```python
from build123d import *

# Parameters (mm, degrees)
SKIZZE1_W                       = 12
SKIZZE1_H                       = 29
SKIZZE1_W_2                     = 15
SKIZZE1_H_2                     = 4
AUFSATZ_LINEAR_AUSTRAGEN1_DEPTH = 4
SKIZZE2_W                       = 1.5
SKIZZE2_H                       = 4
SCHNITT_LINEAR_AUSTRAGEN1_DEPTH = 5
VERRUNDUNG1_R                   = 2


with BuildPart() as part:
    # Skizze1 → Aufsatz-Linear austragen1 (new body)
    with BuildSketch(Plane.XY):
        with Locations((0, -16.5)):
            Rectangle(SKIZZE1_W, SKIZZE1_H)
        Rectangle(SKIZZE1_W_2, SKIZZE1_H_2)
    extrude(amount=AUFSATZ_LINEAR_AUSTRAGEN1_DEPTH)

    # Skizze2 → Schnitt-Linear austragen1 (cut, through all)
    with BuildSketch(Plane.XY.offset(4)):
        with Locations((-5.25, -24)):
            Rectangle(SKIZZE2_W, SKIZZE2_H)
        with Locations((5.25, -24)):
            Rectangle(SKIZZE2_W, SKIZZE2_H)
    extrude(amount=-SCHNITT_LINEAR_AUSTRAGEN1_DEPTH, mode=Mode.SUBTRACT)

    # Verrundung1
    verrundung1_edges = [part.edges().sort_by_distance(p)[0] for p in [
        (6, -31, 2),
        (-6, -31, 2),
    ]]
    fillet(verrundung1_edges, radius=VERRUNDUNG1_R)


solid = part.part
```
Geometry: final body of the model. Coordinates: model frame, mm. A direction names the side the tool comes from. Round coordinates to 2 decimals unless told otherwise and drop trailing zeros. Loops run counter-clockwise (first coordinate to the right, second up) from the corner with the lowest first, then second, coordinate; pieces in that order, holes last.
Item 1: Section B-B, the plane y = -17. Output: boundary loops of the cut face in (x, z).
Checked values:
outline: (-6, 0) - (6, 0) - (6, 4) - (-6, 4) - close
Item 2: Line query: L1, parallel to X at y = -19.5, z = 0.9; L2, parallel to X at y = -24, z = 2.35; L3, parallel to Y at x = -6.5, z = 2.65. Output: solid intervals per line, ascending.
Checked values:
L1: x = -6 to 6
L2: x = -4.5 to 4.5
L3: y = -2 to 2
Item 3: Mould query, pull axis Y, two halves, no side actions, for faces 6 (the flat face through (6, -28, 2)), 7 (the cylindrical face through (5.4, -30.43, 2.03)), 8 (the flat face through (5, -26, 2)). Classes: released by +Y, released by -Y, zero draft, split by the parting line, or undercut.
Checked values:
face 6: zero draft
face 7: released by -Y
face 8: undercut
Item 4: Section A-A, the plane z = 3.2. Output: boundary loops of the cut face in (x, y).
Checked values:
outline: (-7.5, -2) - (-6, -2) - (-6, -22) - (-4.5, -22) - (-4.5, -26) - (-6, -26) - (-6, -29) arc R2 ccw to (-4, -31) - (4, -31) arc R2 ccw to (6, -29) - (6, -26) - (4.5, -26) - (4.5, -22) - (6, -22) - (6, -2) - (7.5, -2) - (7.5, 2) - (-7.5, 2) - close
Item 5: Section C-C, the plane y = -25.5. Output: boundary loops of the cut face in (x, z).
Checked values:
outline: (-4.5, 0) - (4.5, 0) - (4.5, 4) - (-4.5, 4) - close
Item 6: Contact query for flat-ended pins moving along their axis: P1, Ø1.2, axis at y = -11.5, z = 1, coming from the -X side; P2, Ø0.9, axis at y = -27, z = 2.5, coming from the +X side; P3, Ø1.2, axis at y = -23, z = 1.5, coming from the +X side. Output: stop coordinate, or through.
Checked values:
P1: stops at x = -6
P2: stops at x = 6
P3: stops at x = 4.5
Item 7: Reachability of faces 1 (the flat face through (-7, -2, 2)), 2 (the flat face through (-4.5, -24, 2)), 3 (the flat face through (7, -2, 2)), 4 (the flat face through (0, -14, 0)), 5 (the flat face through (4.5, -24, 2)) from +Z, -Z, +X, -X, +Y, -Y: full face, straight path, thin tool, end or side. Return the list, or none.
Checked values:
face 1: +Z, -Z, -X, -Y
face 2: +Z, -Z, -X
face 3: +Z, -Z, +X, -Y
face 4: -Z, +X, -X, +Y, -Y
face 5: +Z, -Z, +X
